Verification items for this drawing (mm, ordinates from the low corner). A direction names the side the tool comes from. Give positions to 0.01 mm unless a question says otherwise; leave off trailing zeros. Loops run counter-clockwise (first coordinate to the right, second up) from the corner with the lowest first, then second, coordinate; pieces in that order, holes last. Notation, with made-up numbers: (-12.5, 59.25) -> (-7.5, 59.25) arc R22 ccw to (-7.5, 91.25) -> close; hole circle Ø2 at (-26, -11). An arc over 180 degrees is marked (long way). Answer as a JSON object with one key per item and string values.
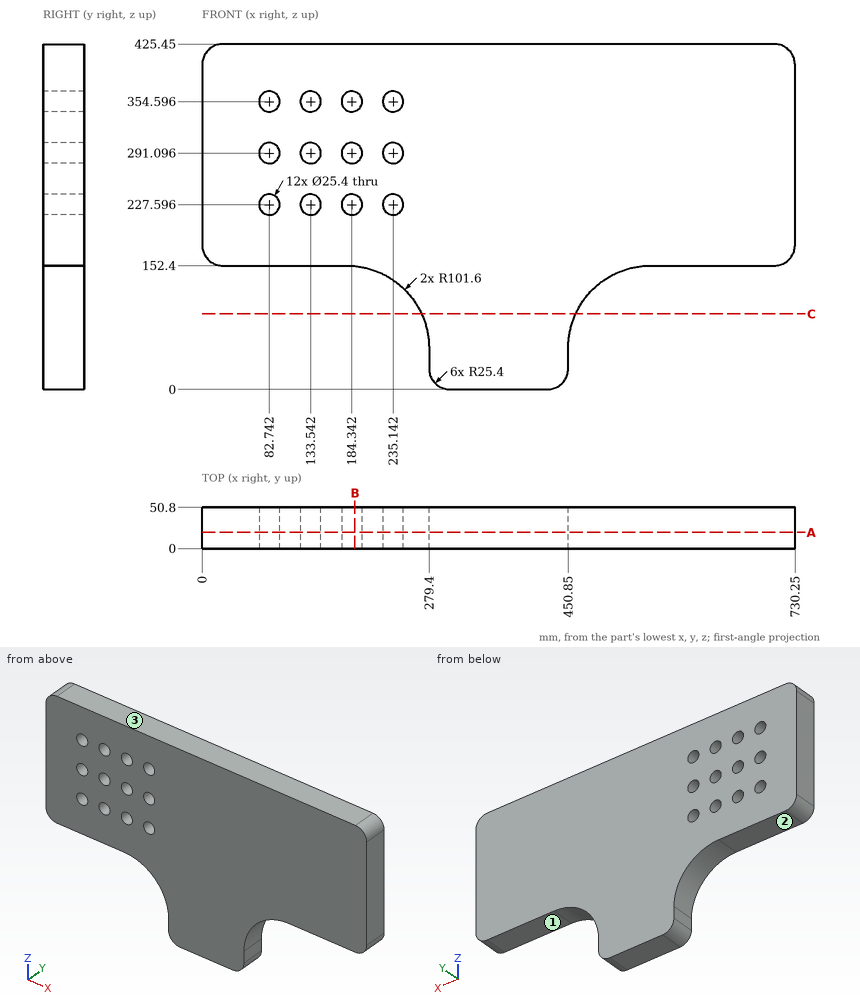
1) Section check A-A on y = 20. Count the separate pieces of the cut face and the enclosed holes in it, plus the area to 3 significant figures.
Geometry check:
{"separate pieces": "1", "enclosed holes": "12", "area": "223,000 mm2"}
2) Material ranges on line 1 along Z through (x, y) = (675.5, 23); line 2 along Z through (x, y) = (189, 38.5); line 3 along X through (y, z) = (18.5, 235.5), recorded low to high. Write a range as from..to.
Geometry check:
{"line 1": "z = 152.4..425.45", "line 2": "z = 151.78..215.78, 239.41..279.28, 302.91..342.78, 366.41..425.45", "line 3": "x = 0..72.8, 92.68..123.6, 143.48..174.4, 194.28..225.2, 245.08..730.25"}
3) Section check B-B on x = 188. Record the cut outline in (y, z).
Geometry check:
{"outline": "(0, 151.89) -> (50.8, 151.89) -> (50.8, 215.43) -> (0, 215.43) -> close; (0, 239.76) -> (50.8, 239.76) -> (50.8, 278.93) -> (0, 278.93) -> close; (0, 303.26) -> (50.8, 303.26) -> (50.8, 342.43) -> (0, 342.43) -> close; (0, 366.76) -> (50.8, 366.76) -> (50.8, 425.45) -> (0, 425.45) -> close"}
4) Depth check by flat-ended pin: P1, Ø15, axis at x = 649.5, y = 32, coming from the -Z side; P2, Ø12, axis at x = 258.5, y = 13.5, coming from the -Z side. Enter the tip coordinate at first touch or a pass-through.
Geometry check:
{"P1": "stops at z = 152.4", "P2": "stops at z = 103.77"}
5) Section check C-C on z = 93. Record the cut outline in (x, y), plus the area to 3 significant figures.
Geometry check:
{"outline": "(270.22, 0) -> (460.03, 0) -> (460.03, 50.8) -> (270.22, 50.8) -> close", "area": "9,640 mm2"}
6) Tool access check on the marked faces 1, 2 and 3. Record the directions out of +Z, -Z, +X, -X, +Y, -Y that give a thin tool (end or side, any length) a straight path to the whole face; none if there is none.
Geometry check:
{"face 1": "-Z, +X, +Y, -Y", "face 2": "-Z, -X, +Y, -Y", "face 3": "+Z, +X, -X, +Y, -Y"}
